Verification items for the finished model (mm, model axes). A direction names the side the tool comes from. Round coordinates to 2 decimals unless told otherwise and drop trailing zeros. Loops run counter-clockwise (first coordinate to the right, second up) from the corner with the lowest first, then second, coordinate; pieces in that order, holes last. Notation, with made-up numbers: (40, 89) -> (98, 89) arc R8 cw to (98, 93) -> close; hole circle Ø7 at (7.5, -34). An arc over 180 degrees is marked (long way). Use CSV: the item, a comma, the result in double quotes. Start each with the question number.
```python
from build123d import *

# Parameters (mm, degrees)
SKETCH1_R           = 1.5
SKETCH1_R_2         = 7
BOSS_EXTRUDE1_DEPTH = 1.5
SKETCH1_3_R         = 13
SKETCH1_3_R_2       = 11
BOSS_EXTRUDE2_DEPTH = 1


with BuildPart() as part:
    # Sketch1 → Boss-Extrude1 (new body)
    with BuildSketch(Plane(origin=(0, 0, 0), x_dir=(1, 0, 0), z_dir=(0, 1, 0))):
        with BuildLine():
            ThreePointArc((14.297039341, 7.182942718), (14.019613784, 8.984050781), (14.849242405, 10.606601718))
            ThreePointArc((14.849242405, 10.606601718), (14.849242405, 14.849242405), (10.606601718, 14.849242405))
            ThreePointArc((10.606601718, 14.849242405), (8.984050781, 14.019613784), (7.182942718, 14.297039341))
            ThreePointArc((7.182942718, 14.297039341), (0, 16), (-7.182942718, 14.297039341))
            ThreePointArc((-7.182942718, 14.297039341), (-8.984050781, 14.019613784), (-10.606601718, 14.849242405))
            ThreePointArc((-10.606601718, 14.849242405), (-14.849242405, 14.849242405), (-14.849242405, 10.606601718))
            ThreePointArc((-14.849242405, 10.606601718), (-14.019613784, 8.984050781), (-14.297039341, 7.182942718))
            ThreePointArc((-14.297039341, 7.182942718), (-16, 0), (-14.297039341, -7.182942718))
            ThreePointArc((-14.297039341, -7.182942718), (-14.019613784, -8.984050781), (-14.849242405, -10.606601718))
            ThreePointArc((-14.849242405, -10.606601718), (-14.849242405, -14.849242405), (-10.606601718, -14.849242405))
            ThreePointArc((-10.606601718, -14.849242405), (-8.984050781, -14.019613784), (-7.182942718, -14.297039341))
            ThreePointArc((-7.182942718, -14.297039341), (0, -16), (7.182942718, -14.297039341))
            ThreePointArc((7.182942718, -14.297039341), (8.984050781, -14.019613784), (10.606601718, -14.849242405))
            ThreePointArc((10.606601718, -14.849242405), (14.849242405, -14.849242405), (14.849242405, -10.606601718))
            ThreePointArc((14.849242405, -10.606601718), (14.019613784, -8.984050781), (14.297039341, -7.182942718))
            ThreePointArc((14.297039341, -7.182942718), (16, 0), (14.297039341, 7.182942718))
        make_face()
        with Locations((12.727922061, 12.727922061)):
            Circle(SKETCH1_R, mode=Mode.SUBTRACT)
        with Locations((12.727922061, -12.727922061)):
            Circle(SKETCH1_R, mode=Mode.SUBTRACT)
        with Locations((-12.727922061, 12.727922061)):
            Circle(SKETCH1_R, mode=Mode.SUBTRACT)
        with Locations((-12.727922061, -12.727922061)):
            Circle(SKETCH1_R, mode=Mode.SUBTRACT)
        Circle(SKETCH1_R_2, mode=Mode.SUBTRACT)
    extrude(amount=BOSS_EXTRUDE1_DEPTH)

    # Sketch1<3> → Boss-Extrude2 (add)
    with BuildSketch(Plane(origin=(0, 0, 0), x_dir=(1, 0, 0), z_dir=(0, 1, 0))):
        Circle(SKETCH1_3_R)
        Circle(SKETCH1_3_R_2, mode=Mode.SUBTRACT)
    extrude(amount=-BOSS_EXTRUDE2_DEPTH)


solid = part.part
```
Q1. Release check for a two-part mould opening along X. For faces 3 (the face through (16, 1, 0)), 4 (the face through (14.8, 0.7, 14.9)), 5 (the face through (-14.016, 0.74, 8.958)), 6 (the face through (-2.38, -0.49, 10.74)) record: +X half, -X half, draft (parallel to the pull), parting line (faces both ways), or undercut.
Q2. Cross-section at B-B (x = 0). Record the boundary of the cut face in (y, z).
Q3. Cross-section at A-A (z = 0). Record the boundary of the cut face in (x, y).
Q4. Cross-section at C-C (x = -10). Record the boundary of the cut face in (y, z).
Q5. Thickness scan on L1, parallel to X at y = -0.2, z = 0; L2, parallel to Y at x = 5.5, z = -5; L3, parallel to X at y = 0.45, z = -13. Record the ranges inside material, lowest first. Write a range as from..to.
Q6. Tool access check on faces 1 (the face through (0, 1, -16)), 2 (the face through (7.2, 0, -0.2)). Record the directions out of +Z, -Z, +X, -X, +Y, -Y that give a thin tool (end or side, any length) a straight path to the whole face; none if there is none.
Q7. Depth check by flat-ended pin: pin 1 Ø1 at (y, z) = (0.5, 10.5) entering from -X; pin 2 Ø1.5 at (y, z) = (0, -5.5) entering from +X; pin 3 Ø4 at (x, z) = (12.73, 12.73) entering from -Y. Enter the tip coordinate at first touch or a pass-through.
Answer list:
1,face 3,"+X half"
1,face 4,"undercut"
1,face 5,"-X half"
1,face 6,"undercut"
2,outline,"(-1, -13) -> (0, -13) -> (0, -16) -> (1.5, -16) -> (1.5, -7) -> (0, -7) -> (0, -11) -> (-1, -11) -> close; (-1, 11) -> (0, 11) -> (0, 7) -> (1.5, 7) -> (1.5, 16) -> (0, 16) -> (0, 13) -> (-1, 13) -> close"
3,outline,"(-16, 0) -> (-13, 0) -> (-13, -1) -> (-11, -1) -> (-11, 0) -> (-7, 0) -> (-7, 1.5) -> (-16, 1.5) -> close; (7, 0) -> (11, 0) -> (11, -1) -> (13, -1) -> (13, 0) -> (16, 0) -> (16, 1.5) -> (7, 1.5) -> close"
4,outline,"(-1, -8.31) -> (0, -8.31) -> (0, -14.38) -> (1.5, -14.38) -> (1.5, 14.38) -> (0, 14.38) -> (0, 8.31) -> (-1, 8.31) -> (-1, 4.58) -> (0, 4.58) -> (0, -4.58) -> (-1, -4.58) -> close"
5,L1,"x = -13..-11, 11..13"
5,L2,"y = 0..1.5"
5,L3,"x = -15.72..-14.2, -11.25..11.25, 14.2..15.72"
6,face 1,"-Z, +Y, -Y"
6,face 2,"-Y"
7,pin 1,"stops at x = -15.18"
7,pin 2,"stops at x = 15.28"
7,pin 3,"stops at y = 0"
